from build123d import *

# Parameters (mm, degrees)
SKETCH1_R           = 2.5
SKETCH1_R_2         = 6
BOSS_EXTRUDE1_DEPTH = 17
SKETCH2_R           = 5
CUT_EXTRUDE1_DEPTH  = 15


with BuildPart() as part:
    # Sketch1 → Boss-Extrude1 (new body)
    with BuildSketch(Plane(origin=(0, 0, 0), x_dir=(1, 0, 0), z_dir=(0, 1, 0))):
        with BuildLine():
            Line((-16, 20), (16, 20))
            Line((16, 20), (16, -10))
            ThreePointArc((16, -10), (13.071067812, -17.071067812), (6, -20))
            Line((6, -20), (-6, -20))
            ThreePointArc((-6, -20), (-13.071067812, -17.071067812), (-16, -10))
            Line((-16, -10), (-16, 20))
        make_face()
        with Locations((0, 12.5)):
            Circle(SKETCH1_R, mode=Mode.SUBTRACT)
        with Locations((0, -5)):
            Circle(SKETCH1_R_2, mode=Mode.SUBTRACT)
    extrude(amount=BOSS_EXTRUDE1_DEPTH)

    # Sketch2 → Cut-Extrude1 (cut)
    with BuildSketch(Plane(origin=(0, 0, -20), x_dir=(-1, 0, 0), z_dir=(0, 0, -1))):
        with Locations((0, 8.5)):
            Circle(SKETCH2_R)
    extrude(amount=-CUT_EXTRUDE1_DEPTH, mode=Mode.SUBTRACT)


solid = part.part
Here's how the part is built. I have some questions about the finished solid (model axes, mm). A direction names the side the tool comes from. Give positions to 0.01 mm unless a question says otherwise; leave off trailing zeros. Loops run counter-clockwise (first coordinate to the right, second up) from the corner with the lowest first, then second, coordinate; pieces in that order, holes last. Notation, with made-up numbers: (46, 16.25) -> (95, 16.25) arc R11 ccw to (95, 29.25) -> close; hole circle Ø3 at (-40, 83.25). An arc over 180 degrees is marked (long way). Answer as a JSON object with one key per item and string values. Group by question number.
Item 1: Imagine slicing it at A-A on z = 5. Write out the boundary of the cut face in (x, y), then the cut area to 3 significant figures.
Item 2: Imagine slicing it at D-D on z = -6.5. Write out the boundary of the cut face in (x, y), then the cut area to 3 significant figures.
Item 3: Imagine slicing it at C-C on y = 8.5. Write out the boundary of the cut face in (x, z).
Item 4: Thinking about a two-plate mould opening in Z: for faces 3 (the flat face through (0, 9, -5)), 4 (the flat face through (0, 0, -5)), 5 (the cylindrical face through (-12.99, 8.38, 17.15)), 6 (the cylindrical face through (2.31, 14.89, -11.54)), which applies, pulls with the +Z half, pulls with the -Z half, needs draft (parallel to the pull), parting line crosses it, or undercut?
Item 5: On a 3-axis mill with a long thin cutter (end or side, diameter ignored), from which of +Z, -Z, +X, -X, +Y, -Y can I reach the whole of each face in a straight line? I mean faces 1 (the cylindrical face through (-0.54, 2.06, -10.06)), 2 (the cylindrical face through (-2.688, 12.716, -12.605)). Say none if no direction works.
Item 6: I need wall thicknesses on L1, parallel to Z at x = 0, y = 14.85; L2, parallel to Z at x = 0, y = 7.25; L3, parallel to X at y = 14.95, z = -12.5. Which ranges of each line are inside material? Lowest first, please.
Item 7: Will these pins go through, and if not, where does the flat tip stop? pin 1 (15.5 mm diameter, centred on x = 0, z = 5, fed in from +Y); pin 2 (2 mm diameter, centred on x = 8.5, y = 13, fed in from +Z); pin 3 (2 mm diameter, centred on x = 0, y = 9.5, fed in from -Z); pin 4 (4 mm diameter, centred on x = 12, y = 3, fed in from +Z).
Item 8: Imagine slicing it at B-B on x = 0. Write out the boundary of the cut face in (y, z).
Answer list:
{
 "1": {"outline": "(-16, 0) -> (-6, 0) -> (-6, 17) -> (-16, 17) -> close; (6, 0) -> (16, 0) -> (16, 17) -> (6, 17) -> close", "area": "340 mm2"},
 "2": {"outline": "(-16, 0) -> (16, 0) -> (16, 17) -> (-16, 17) -> close; hole circle Ø10 at (0, 8.5)", "area": "465 mm2"},
 "3": {"outline": "(-16, -20) -> (-5, -20) -> (-5, -5) -> (5, -5) -> (5, -20) -> (16, -20) -> (16, 10) arc R10 ccw to (6, 20) -> (-6, 20) arc R10 ccw to (-16, 10) -> close; hole circle Ø12 at (0, 5)"},
 "4": {"face 3": "pulls with the -Z half", "face 4": "needs draft", "face 5": "pulls with the +Z half", "face 6": "undercut"},
 "5": {"face 1": "+Y, -Y", "face 2": "-Z"},
 "6": {"L1": "z = -20 to -15, -10 to -1, 11 to 20", "L2": "z = -5 to -1, 11 to 20", "L3": "x = -16 to -2.5, 2.5 to 16"},
 "7": {"pin 1": "stops at y = 17", "pin 2": "stops at z = 19.89", "pin 3": "stops at z = -5", "pin 4": "stops at z = 19.17"},
 "8": {"outline": "(0, -20) -> (3.5, -20) -> (3.5, -15) -> (0, -15) -> close; (0, -10) -> (3.5, -10) -> (3.5, -5) -> (13.5, -5) -> (13.5, -10) -> (17, -10) -> (17, -1) -> (0, -1) -> close; (0, 11) -> (17, 11) -> (17, 20) -> (0, 20) -> close; (13.5, -20) -> (17, -20) -> (17, -15) -> (13.5, -15) -> close"}
}
